from build123d import *

# Parameters (mm, degrees)
BOSS_EXTRUDE1_DEPTH = 40.1
SKETCH3_R           = 1.35
CUT_EXTRUDE2_DEPTH  = 50.8
SKETCH4_R           = 1.016
CUT_EXTRUDE3_DEPTH  = 50.8
SKETCH6_W           = 62.086073973
SKETCH6_H           = 34.1
CUT_EXTRUDE4_DEPTH  = 6
BOSS_EXTRUDE5_DEPTH = 2
FILLET1_R           = 1
SKETCH17_W          = 87.972052268
SKETCH17_H          = 62.392444702
CUT_EXTRUDE5_DEPTH  = 101.73954578
SKETCH18_W          = 11.938
SKETCH18_H          = 8.5
CUT_EXTRUDE6_DEPTH  = 87.3496381
SKETCH19_W          = 9.553882118
SKETCH19_H          = 7.100488973
BOSS_EXTRUDE6_DEPTH = 40
SKETCH20_W          = 8.332283041
SKETCH20_H          = 7.273954642
CUT_EXTRUDE8_DEPTH  = 87.3496381
FILLET2_R           = 7
SKETCH21_W          = 4.7244
SKETCH21_H          = 10
CUT_EXTRUDE9_DEPTH  = 87.3496381
SKETCH22_W          = 34.1
SKETCH22_H          = 6
CUT_EXTRUDE10_DEPTH = 69.201135731


with BuildPart() as part:
    # Sketch1 → Boss-Extrude1 (new body)
    with BuildSketch(Plane.XY):
        Polygon((0, 0), (0, 52.578), (6, 52.578), (6, 8.5), (76, 8.5), (76, 0), align=None)
    extrude(amount=BOSS_EXTRUDE1_DEPTH)

    # Sketch3 → Cut-Extrude2 (cut)
    with BuildSketch(Plane.XY.offset(40.1)):
        with Locations((27.996, 2.8)):
            Circle(SKETCH3_R)
        with Locations((49.996, 2.8)):
            Circle(SKETCH3_R)
        with Locations((71.996, 2.8)):
            Circle(SKETCH3_R)
    extrude(amount=-CUT_EXTRUDE2_DEPTH, mode=Mode.SUBTRACT)

    # Sketch4 → Cut-Extrude3 (cut)
    with BuildSketch(Plane.ZY):
        with Locations((27.88, 17.6)):
            Circle(SKETCH4_R)
        with Locations(Location((11.88, 17.6, 0), (0, 0, 270))):
            Circle(SKETCH4_R)
        with Locations((27.88, 49.6)):
            Circle(SKETCH4_R)
        with Locations(Location((11.88, 49.6, 0), (0, 0, 270))):
            Circle(SKETCH4_R)
    extrude(amount=-CUT_EXTRUDE3_DEPTH, mode=Mode.SUBTRACT)

    # Sketch6 → Cut-Extrude4 (cut)
    with BuildSketch(Plane.XZ):
        with Locations((50.043036987, 20.05)):
            Rectangle(SKETCH6_W, SKETCH6_H)
    extrude(amount=-CUT_EXTRUDE4_DEPTH, mode=Mode.SUBTRACT)

    # Sketch16 → Boss-Extrude5 (add)
    with BuildSketch(Plane.XY.offset(40.1)):
        Polygon((6, 8.5), (26, 8.5), (6, 33.5), align=None)
    boss_extrude5 = extrude(amount=-BOSS_EXTRUDE5_DEPTH)

    # Mirror2: Boss-Extrude5 across plane
    add(boss_extrude5.mirror(Plane(origin=(0, 0, 20.05), x_dir=(1, 0, 0), z_dir=(0, 0, -1))))

    # Fillet1
    fillet1_edges = [part.edges().sort_by_distance(p)[0] for p in [
        (0, 0, 20.05),
        (76, 0, 38.6),
        (3, 52.578, 40.1),
        (76, 0, 1.5),
        (3, 52.578, 0),
    ]]
    fillet(fillet1_edges, radius=FILLET1_R)

    # Sketch17 → Cut-Extrude5 (cut, through all)
    with BuildSketch(Plane.XY.offset(40.1)):
        with Locations((43.986026134, 39.696222351)):
            Rectangle(SKETCH17_W, SKETCH17_H)
    extrude(amount=-CUT_EXTRUDE5_DEPTH, mode=Mode.SUBTRACT)

    # Sketch18 → Cut-Extrude6 (cut, through all)
    with BuildSketch(Plane.XY.offset(40.1)):
        with Locations((5.969, 4.25)):
            Rectangle(SKETCH18_W, SKETCH18_H)
    extrude(amount=-CUT_EXTRUDE6_DEPTH, mode=Mode.SUBTRACT)

    # Sketch19 → Boss-Extrude6 (add)
    with BuildSketch(Plane.XY.offset(40.1)):
        with Locations((16.714941059, 3.550244487)):
            Rectangle(SKETCH19_W, SKETCH19_H)
    extrude(amount=-BOSS_EXTRUDE6_DEPTH)

    # Sketch20 → Cut-Extrude8 (cut, through all)
    with BuildSketch(Plane.XY.offset(40.1)):
        with Locations((16.104141521, 3.636977321)):
            Rectangle(SKETCH20_W, SKETCH20_H)
    extrude(amount=-CUT_EXTRUDE8_DEPTH, mode=Mode.SUBTRACT)

    # Fillet2
    fillet2_edges = [part.edges().sort_by_distance(p)[0] for p in [
        (20.270283041, 7.273954642, 20.05),
    ]]
    fillet(fillet2_edges, radius=FILLET2_R)

    # Sketch21 → Cut-Extrude9 (cut, through all)
    with BuildSketch(Plane.XY.offset(40.1)):
        with Locations((14.3002, 3.5)):
            Rectangle(SKETCH21_W, SKETCH21_H)
    extrude(amount=-CUT_EXTRUDE9_DEPTH, mode=Mode.SUBTRACT)

    # Sketch22 → Cut-Extrude10 (cut, through all)
    with BuildSketch(Plane(origin=(21.491882118, 0, 0), x_dir=(0, 0, -1), z_dir=(1, 0, 0))):
        with Locations((-20.05, 3)):
            Rectangle(SKETCH22_W, SKETCH22_H)
    extrude(amount=-CUT_EXTRUDE10_DEPTH, mode=Mode.SUBTRACT)


solid = part.part
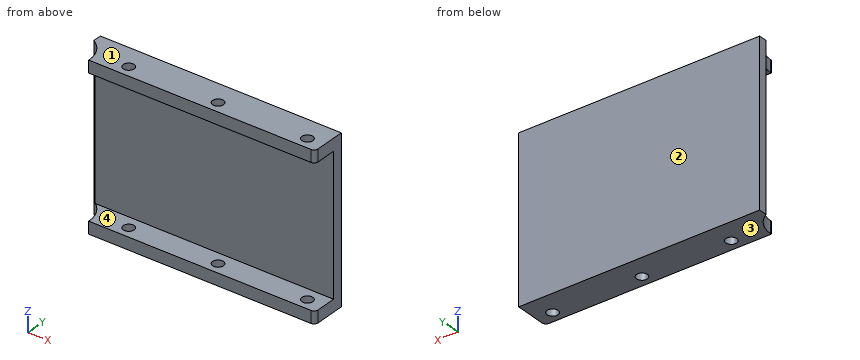
Model file for the job. Use its own axes, mm. Face numbers are marked on the shaded views. Coordinates: 2 decimals unless noted, no trailing zeros. Loops run counter-clockwise (first coordinate to the right, second up) from the corner with the lowest first, then second, coordinate; pieces in that order, holes last. Notation, with made-up numbers: (14, 34.5) -> (32, 34.5) arc R19 ccw to (32, 44.5) -> close; hole circle Ø10 at (24, -20.75). An arc over 180 degrees is marked (long way). Use one line per item in the form item = value. Start each with the question number.
(1) Pull direction Z, two halves, no side cores. Call the marked faces 1, 2, 3 and 4: pulls with the +Z half, pulls with the -Z half, needs draft (parallel to the pull), parting line crosses it, or undercut.
(2) Probe probe 1 along Y at (x, z) = (34, 19.5); probe 2 along Z at (x, y) = (50, 1). List the from-to ranges inside material, lowest first. Write a range as from..to.
(3) Cut at C-C on x = 62. Give the cut face in (y, z).
(4) Cut at B-B on z = 2. Give the cut face in (x, y), and give its area (3 significant figures).
(5) Cut at A-A on y = 2.8. Give the number of separate pieces and of enclosed holes in the cut face, and give its area (3 significant figures).
(6) Cut at D-D on z = 15.5. Give the cut face in (x, y), and give its area (3 significant figures).
(7) Flat gauge pins, fed straight in: pin 1 (1.6 mm diameter, centred on x = 27.996, y = 2.8, fed in from -Z); pin 2 (17 mm diameter, centred on x = 60.5, z = 15.5, fed in from -Y). Where does each tip first touch, or does it go through?
Values:
q1.face_1 = pulls with the +Z half
q1.face_2 = needs draft
q1.face_3 = pulls with the -Z half
q1.face_4 = undercut
q2.probe_1 = 6..8.5
q2.probe_2 = 0..3, 37.1..40.1
q3.outline = (0, 0) -> (8.5, 0) -> (8.5, 40.1) -> (0, 40.1) -> (0, 37.1) -> (6, 37.1) -> (6, 3) -> (0, 3) -> close
q4.outline = (16.66, 6.4) arc R7 cw to (20.27, 0.27) -> (20.27, 0) -> (75, 0) arc R1 ccw to (76, 1) -> (76, 8.5) -> (16.66, 8.5) -> close; hole circle Ø2.7 at (28, 2.8); hole circle Ø2.7 at (50, 2.8); hole circle Ø2.7 at (72, 2.8)
q4.area = 470 mm2
q5.separate_pieces = 8
q5.enclosed_holes = 0
q5.area = 289 mm2
q6.outline = (16.66, 6.4) arc R7 cw to (17.3, 6) -> (76, 6) -> (76, 8.5) -> (16.66, 8.5) -> close
q6.area = 148 mm2
q7.pin_1 = through
q7.pin_2 = 6
